Autodesk Inventor part; units mm, degrees
ref_plane "YZ Plane" through (0, 0, 0) normal (1, 0, 0) x (0, 1, 0)
ref_plane "XZ Plane" through (0, 0, 0) normal (0, 1, 0) x (-1, 0, 0)
ref_plane "XY Plane" through (0, 0, 0) normal (0, 0, 1) x (1, 0, 0)
sketch "Esboço1" plane through (0, 0, 0) normal (0, 1, 0) x (-1, 0, 0)
  line L0 (-20, 20) -> (20, 20)
  line L1 (20, 20) -> (20, -20)
  line L2 (20, -20) -> (-20, -20)
  line L3 (-20, -20) -> (-20, 20)
  point P0 (0, 0)
extrude "Extrusão1" add sketch "Esboço1" along normal mid plane 5
sketch "Esboço3" plane through (0, 2.5, 0) normal (0, 1, 0) x (1, 0, 0)
  circle A0 centre (0, 0) radius 5
  circle A1 centre (0, 0) radius 4
  dimension "d13" = 10
  dimension "d14" = 8
extrude "Extrusão2" add sketch "Esboço3" along normal blind 7.5 contours A0 | A1
chamfer "Chanfro1" distance 1 angle 45 1 edges at (-5, 10, 0)
properties part number "peça1_trabalho2"
Model file for the job. Use its own axes, mm. A direction names the side the tool comes from. Give positions to 0.01 mm unless a question says otherwise; leave off trailing zeros. Loops run counter-clockwise (first coordinate to the right, second up) from the corner with the lowest first, then second, coordinate; pieces in that order, holes last. Notation, with made-up numbers: (60.5, 37) - (66.5, 37) arc R18 cw to (66.5, 54) - close; hole circle Ø1 at (62, 47.5). An arc over 180 degrees is marked (long way). One line per item, written item: value. Start each with the question number.
1. Slice it at A-A (z = 0). List the corners of the cut face in (x, y), plus the area to 3 significant figures.
2. Probe L1, parallel to Y at x = 16, z = -15.5; L2, parallel to Z at x = -4.5, y = 3.75; L3, parallel to X at y = 3, z = -2. List the from-to ranges inside material, lowest first. Write a range as from..to.
3. Which spindle directions (+Z, -Z, +X, -X, +Y, -Y) get a long thin tool onto all of the face, cutting with end or side? Do faces 1 (the cylindrical face through (-1.08, 5.7, -4.88)), 2 (the flat face through (0, 0, -20)). Say none if no direction does.
4. Slice it at C-C (y = 8.25). List the corners of the cut face in (x, z).
5. Pin check, flat tips, straight feed: pin 1 (4 mm diameter, centred on y = 7, z = 3.5, fed in from -X); pin 2 (5 mm diameter, centred on x = 6, y = 7.5, fed in from +Z); pin 3 (1 mm diameter, centred on y = 4, z = 3, fed in from +X). Stop position of each tip, or through.
6. Slice it at D-D (x = 14). List the corners of the cut face in (y, z), plus the area to 3 significant figures.
7. Slice it at B-B (x = 0). List the corners of the cut face in (y, z), plus the area to 3 significant figures.
Solution:
1. outline: (-20, -2.5) - (20, -2.5) - (20, 2.5) - (5, 2.5) - (5, 9) - (4, 10) - (-4, 10) - (-5, 9) - (-5, 2.5) - (-20, 2.5) - close
1. area: 274 mm^2
2. L1: y = -2.5..2.5
2. L2: z = -2.18..2.18
2. L3: x = -4.58..4.58
3. face 1: +Y
3. face 2: -Z, +X, -X, +Y, -Y
4. outline: circle Ø10 at (0, 0)
5. pin 1: stops at x = -4.77
5. pin 2: stops at z = 3.57
5. pin 3: stops at x = 4.33
6. outline: (-2.5, -20) - (2.5, -20) - (2.5, 20) - (-2.5, 20) - close
6. area: 200 mm^2
7. outline: (-2.5, -20) - (2.5, -20) - (2.5, -5) - (9, -5) - (10, -4) - (10, 4) - (9, 5) - (2.5, 5) - (2.5, 20) - (-2.5, 20) - close
7. area: 274 mm^2
